```python
from build123d import *

# Parameters (mm, degrees)
SKETCH_1_W          = 75
SKETCH_1_H          = 15
EXTRUDE_1_DEPTH     = 2
FILLET_1_R          = 7.5
SKETCH_2_R          = 4.5
CUT_EXTRUDE_1_DEPTH = 2
CUT_EXTRUDE_2_DEPTH = 10
FILLET_2_R          = 1


with BuildPart() as part:
    # 草图1 → 凸台-拉伸1 (new body)
    with BuildSketch(Plane.XY):
        Rectangle(SKETCH_1_W, SKETCH_1_H)
    extrude(amount=EXTRUDE_1_DEPTH)

    # 圆角1
    fillet_1_edges = [part.edges().sort_by_distance(p)[0] for p in [
        (37.5, -7.5, 1),
        (-37.5, -7.5, 1),
        (-37.5, 7.5, 1),
        (37.5, 7.5, 1),
    ]]
    fillet(fillet_1_edges, radius=FILLET_1_R - 0.0001)  # a hair under: the kernel refuses the full size

    # 草图2 → 切除-拉伸1 (cut)
    with BuildSketch(Plane.XY.offset(2)):
        with Locations((30, 0)):
            Circle(SKETCH_2_R)
        with Locations((-30, 0)):
            Circle(SKETCH_2_R)
    extrude(amount=-CUT_EXTRUDE_1_DEPTH, mode=Mode.SUBTRACT)

    # 草图3 → 切除-拉伸2 (cut)
    with BuildSketch(Plane.XY.offset(2)):
        Polygon((4.123105626, 0), (20, 3.969223594), (20, -3.969223594), align=None)
        Polygon((-15.876894374, 5), (0, 1.030776406), (15.876894374, 5), align=None)
        Polygon((0, -1.030776406), (15.876894374, -5), (-15.876894374, -5), align=None)
        Polygon((-20, 3.969223594), (-20, -3.969223594), (-4.123105626, 0), align=None)
    extrude(amount=-CUT_EXTRUDE_2_DEPTH, mode=Mode.SUBTRACT)

    # 圆角2
    fillet_2_edges = [part.edges().sort_by_distance(p)[0] for p in [
        (4.123105626, 0, 1),
        (20, 3.969223594, 1),
        (20, -3.969223594, 1),
        (0, -1.030776406, 1),
        (15.876894374, -5, 1),
        (-15.876894374, -5, 1),
        (-20, -3.969223594, 1),
        (-20, 3.969223594, 1),
        (-4.123105626, 0, 1),
        (0, 1.030776406, 1),
        (-15.876894374, 5, 1),
        (15.876894374, 5, 1),
    ]]
    fillet(fillet_2_edges, radius=FILLET_2_R)


solid = part.part
```
Can you work these out from the model? Positions are in its coordinate system, mm. A direction names the side the tool comes from. Give positions to 0.01 mm unless a question says otherwise; leave off trailing zeros. Order: outer loops, then holes, each group sorted by start corner. A loop starts at its lowest first (then second) coordinate and runs counter-clockwise, first axis right, second up. Notation, with made-up numbers: (76, -14.5) - (108, -14.5) arc R29 cw to (108, 18.5) - close; hole circle Ø8 at (-5, 23.25). An arc over 180 degrees is marked (long way). Use a Markdown table: item, result. Add a question column.
Q1. If we section it at B-B on y = -6: Write out the boundary of the cut face in (x, z), plus the area to 3 significant figures.
Q2. If we section it at A-A on z = 0.65: Count the separate pieces of the cut face and the enclosed holes in it, plus the area to 3 significant figures.
Q3. If we mould it in two halves opening along Y, with no side actions, what happens to faces 3 (the cylindrical face through (35.245, -5.361, 1.014)), 4 (the cylindrical face through (35.361, 5.245, 1.014)), 5 (the cylindrical face through (19.61, -3.48, 0.99))? For each: released by +Y, released by -Y, zero draft, split by the parting line, or undercut.
Q4. Please list where these lines run through material, in increasing order: line 1 along Y through (x, z) = (-30, 1.2); line 2 along Y through (x, z) = (-8, 1.3).
Q5. On a 3-axis mill with a long thin cutter (end or side, diameter ignored), from which of +Z, -Z, +X, -X, +Y, -Y can I reach the whole of each face in a straight line? I mean faces 1 (the flat face through (0, -7.5, 1)), 2 (the flat face through (0, -5, 1)). Say none if no direction works.
Answers follow:
| question | item | result |
|---|---|---|
| 1 | outline | (-34.5, 0) - (34.5, 0) - (34.5, 2) - (-34.5, 2) - close |
| 1 | area | 138 mm^2 |
| 2 | separate pieces | 1 |
| 2 | enclosed holes | 6 |
| 2 | area | 731 mm^2 |
| 3 | face 3 | released by -Y |
| 3 | face 4 | released by +Y |
| 3 | face 5 | undercut |
| 4 | line 1 | y = -7.5 to -4.5, 4.5 to 7.5 |
| 4 | line 2 | y = -7.5 to -4.97, -3.03 to -0.97, 0.97 to 3.03, 4.97 to 7.5 |
| 5 | face 1 | +Z, -Z, +X, -X, -Y |
| 5 | face 2 | +Z, -Z |
